Could you check a few things on this model? Use its own coordinates, in mm. A direction names the side the tool comes from. Coordinates: 2 decimals unless noted, no trailing zeros. Loops run counter-clockwise (first coordinate to the right, second up) from the corner with the lowest first, then second, coordinate; pieces in that order, holes last.
from build123d import *

# Parameters (mm, degrees)
BLANKSKE_W          = 127
BLANKSKE_H          = 43.18
BLANK_DEPTH         = 10.16
TOOTHCUTSIM_DEPTH   = 135.524116797
TEETHCUTS_COUNT     = 9
TEETHCUTS_PITCH     = 15.959290662
SKETCH4_R           = 3.175
CUT_EXTRUDE2_DEPTH  = 135.524116797
SKETCH1_W           = 10.16
SKETCH1_H           = 10.16
BOSS_EXTRUDE1_DEPTH = 5.715
SKETCH5_R           = 4.7625
CUT_EXTRUDE3_DEPTH  = 135.524116797


with BuildPart() as part:
    # BlankSke → Blank (new body)
    with BuildSketch(Plane.XY):
        with Locations((63.5, 21.59)):
            Rectangle(BLANKSKE_W, BLANKSKE_H)
    extrude(amount=-BLANK_DEPTH)

    # TooCutSkeSim → ToothCutSim (cut, through all)
    with BuildSketch(Plane.XY):
        Polygon((2.250111678, 31.75), (-2.250111678, 31.75), (-6.4195363, 43.2054), (6.4195363, 43.2054), align=None)
    toothcutsim = extrude(amount=-TOOTHCUTSIM_DEPTH, mode=Mode.SUBTRACT)

    # TeethCuts: ToothCutSim ×9
    with Locations(*[(i * TEETHCUTS_PITCH, 0, 0) for i in range(1, TEETHCUTS_COUNT)]):
        add(toothcutsim, mode=Mode.SUBTRACT)

    # Sketch4 → Cut-Extrude2 (cut, through all)
    with BuildSketch(Plane.ZY):
        with Locations((-5.08, 19.05)):
            Circle(SKETCH4_R)
    extrude(amount=-CUT_EXTRUDE2_DEPTH, mode=Mode.SUBTRACT)

    # Sketch1 → Boss-Extrude1 (add)
    with BuildSketch(Plane.XZ):
        with Locations((5.08, -5.08)):
            Rectangle(SKETCH1_W, SKETCH1_H)
        with Locations((121.92, -5.08)):
            Rectangle(SKETCH1_W, SKETCH1_H)
    extrude(amount=BOSS_EXTRUDE1_DEPTH)

    # Sketch5 → Cut-Extrude3 (cut, through all)
    with BuildSketch(Plane.XY):
        with Locations((63.5, 12.7)):
            Circle(SKETCH5_R)
    extrude(amount=-CUT_EXTRUDE3_DEPTH, mode=Mode.SUBTRACT)


solid = part.part
(1) For pin 1 (0.7 mm diameter, centred on x = 0.5, z = -7, fed in from +Y); pin 2 (3 mm diameter, centred on x = 31.5, z = -7, fed in from -Y), each with a flat end and sliding along its axis, tell me the tip position at first contact or that it passes through.
Answers:
pin 1: stops at y = 31.75
pin 2: stops at y = 0
(2) Imagine slicing it at D-D, the plane x = 104. Write out the boundary of the cut face in (y, z) (3 decimals), and give its area (3 significant figures).
Answers:
outline: (0, -10.16) - (43.18, -10.16) - (43.18, 0) - (0, 0) - close; hole circle Ø6.35 at (19.05, -5.08)
area: 407 mm2
(3) Which directions (+Z, -Z, +X, -X, +Y, -Y) give clear straight access to the entire face, cutting with the end or side of a thin tool? Please do faces 4 (the face through (52.24, 37.55, -5.01)), 5 (the face through (56, 43.18, -5)), 6 (the face through (116.84, -3, -5)).
Answers:
face 4: +Z, -Z, +Y
face 5: +Z, -Z, +X, -X, +Y
face 6: +Z, -Z, -Y
(4) Imagine slicing it at A-A, the plane y = 19.05. Write out the boundary of the cut face in (x, z) (3 decimals).
Answers:
outline: (0, -10.16) - (127, -10.16) - (127, -8.255) - (0, -8.255) - close; (0, -1.905) - (127, -1.905) - (127, 0) - (0, 0) - close
(5) I need wall thicknesses on probe 1 along Y at (x, z) = (71, -5.08) (3 decimals); probe 2 along Y at (x, z) = (81, -3.5); probe 3 along Y at (x, z) = (33, -8.5). Which ranges of each line are inside material? Lowest first, please.
Answers:
probe 1: y = 0 to 15.875, 22.225 to 43.18
probe 2: y = 0 to 16.3, 21.8 to 31.75
probe 3: y = 0 to 31.75
(6) We'd pull the mould along X, two halves only. Please class faces 1 (the face through (84.156, 37.545, -5.009)), 2 (the face through (40, 43.18, -5)), 3 (the face through (63, 0, -5)): +X half, -X half, draft (parallel to the pull), parting line (faces both ways), or undercut.
Answers:
face 1: undercut
face 2: draft
face 3: undercut
(7) Imagine slicing it at B-B, the plane y = 12.7. Write out the boundary of the cut face in (x, z).
Answers:
outline: (0, -10.16) - (58.74, -10.16) - (58.74, 0) - (0, 0) - close; (68.26, -10.16) - (127, -10.16) - (127, 0) - (68.26, 0) - close
